Study the drawing (mm; zero at the part's minimum x, y, z) and answer. A direction names the side the tool comes from. Round coordinates to 2 decimals unless told otherwise and drop trailing zeros. Loops run counter-clockwise (first coordinate to the right, second up) from the corner with the lowest first, then second, coordinate; pieces in that order, holes last. Notation, with made-up numbers: (17, 61) - (42, 61) arc R18 ccw to (42, 95) - close; hole circle Ø11 at (89, 37.5). An arc over 180 degrees is marked (long way). One line per item, written item: value.
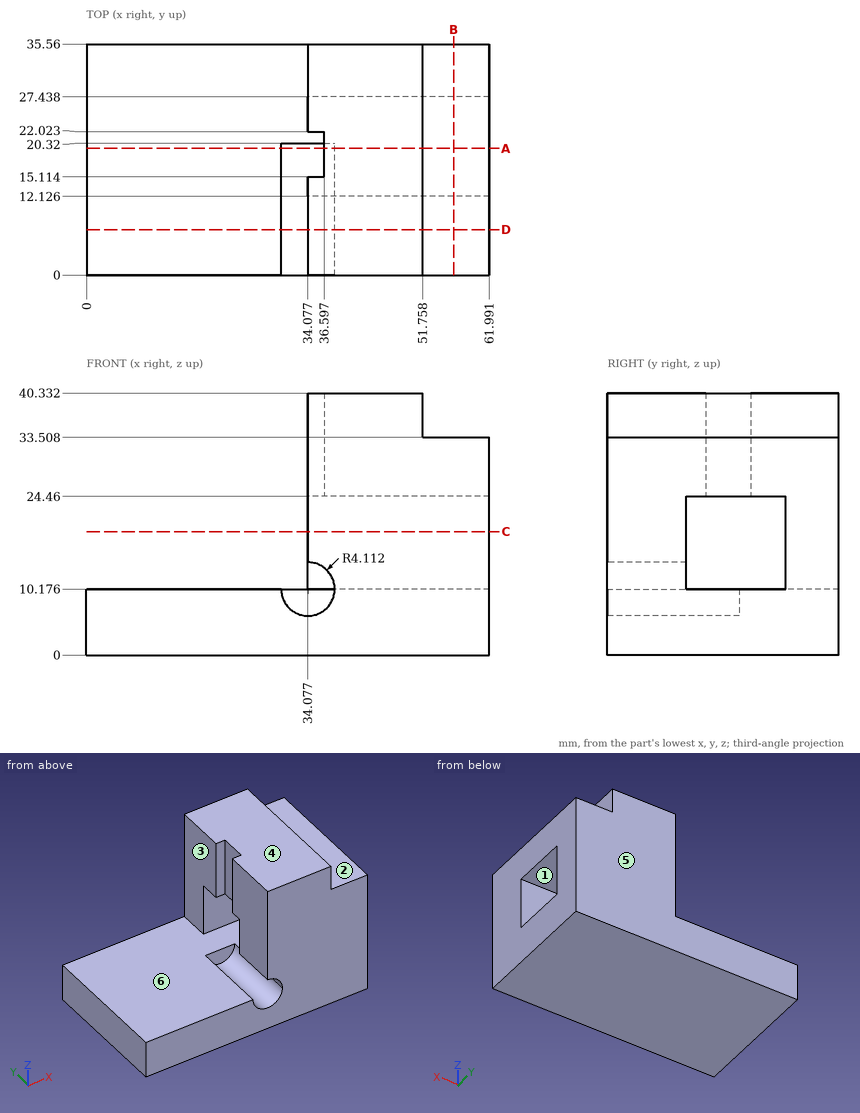
1) A cutting plane is placed at B-B on x = 56.5. Give the vertices of the cut face in (y, z).
Final values:
outline: (0, 0) - (35.56, 0) - (35.56, 33.51) - (0, 33.51) - close; hole (12.13, 10.18) - (27.44, 10.18) - (27.44, 24.46) - (12.13, 24.46) - close
2) Each of these flat-tipped pins is pushed along its axis until it touches: pin 1 Ø4 at (y, z) = (26, 27) entering from -X; pin 2 Ø5.5 at (y, z) = (18, 31) entering from -X; pin 3 Ø8 at (x, y) = (58.5, 12) entering from +Z; pin 4 Ø4 at (y, z) = (19, 21) entering from +X. Where does it stop, or does it pass through?
Final values:
pin 1: x = 34.08
pin 2: x = 36.6
pin 3: z = 33.51
pin 4: through
3) For the marked faces 1, 2 and 3, determine the directions among +Z, -Z, +X, -X, +Y, -Y from which every point of the face is accessible in a straight line to the end or side of a thin tool.
Final values:
face 1: +X, -X
face 2: +Z, +X, +Y, -Y
face 3: +Z, -X, +Y, -Y
4) Consider L1, parallel to Y at x = 52.5, z = 16; L2, parallel to Z at x = 43.5, y = 13; L3, parallel to X at y = 17, z = 37. Determine where each line is inside the solid, lowest interval first.
Final values:
L1: 0 to 12.13, 27.44 to 35.56
L2: 0 to 10.18, 24.46 to 40.33
L3: 36.6 to 51.76
5) A cutting plane is placed at D-D on y = 7. Give the vertices of the cut face in (x, z) (1 decimal).
Final values:
outline: (0, 0) - (62, 0) - (62, 33.5) - (51.8, 33.5) - (51.8, 40.3) - (34.1, 40.3) - (34.1, 14.3) arc R4.1 cw (long way) to (30, 10.2) - (0, 10.2) - close
6) For a pull along Y with two mould halves and no side action, classify the marked faces 4, 5 and 6 as released by +Y, released by -Y, zero draft, split by the parting line, or undercut.
Final values:
face 4: zero draft
face 5: released by +Y
face 6: undercut
7) A cutting plane is placed at A-A on y = 19.5. Give the vertices of the cut face in (x, z) (1 decimal).
Final values:
outline: (0, 0) - (62, 0) - (62, 10.2) - (38.2, 10.2) arc R4.1 cw to (30, 10.2) - (0, 10.2) - close; (36.6, 24.5) - (62, 24.5) - (62, 33.5) - (51.8, 33.5) - (51.8, 40.3) - (36.6, 40.3) - close
8) A cutting plane is placed at C-C on z = 19. Give the vertices of the cut face in (x, y), and give its area (3 significant figures).
Final values:
outline: (34.08, 0) - (61.99, 0) - (61.99, 12.13) - (34.08, 12.13) - close; (34.08, 27.44) - (61.99, 27.44) - (61.99, 35.56) - (34.08, 35.56) - close
area: 565 mm2
